Build history of the part. All positions in model axes, mm. A direction names the side the tool comes from. Round coordinates to 2 decimals unless told otherwise and drop trailing zeros. Write each loop counter-clockwise with the first axis right and the second up, starting at its lowest first coordinate (ties: lowest second). Pieces come first, ordered by that corner, then holes. Notation, with made-up numbers: (28.5, 10.25) - (60.5, 10.25) arc R14 cw to (60.5, 14.25) - close; hole circle Ø8 at (81, 77). An arc over 180 degrees is marked (long way). Answer as a JSON object with one key per item and string values. Group by question number.
Item 1: Probe line 1 (Z direction, x = 22.5, y = 9.1); line 2 (Y direction, x = 26.25, z = -27) (3 decimals); line 3 (Z direction, x = 23.5, y = 8.5). List the from-to ranges inside material, lowest first. Write a range as from..to.
Item 2: Two-plate mould, pull along Y, no slides. Class faces 4 (the flat face through (23.946, 16.896, -28.319)), 5 (the cylindrical face through (23.95, 10.18, -28.18)), 6 (the flat face through (24, 9, -35)): +Y half, -Y half, draft (parallel to the pull), parting line (faces both ways), or undercut.
Item 3: Flat gauge pin, fed straight in: pin 1 (0.7 mm diameter, centred on x = 22.5, z = -35, fed in from +Y). Where does the tip first touch, or does it go through?
Item 4: Slice it at A-A, the plane z = -27. List the corners of the cut face in (x, y) (3 decimals), then the cut area to 3 significant figures.
Item 5: Which spindle directions (+Z, -Z, +X, -X, +Y, -Y) get a long thin tool onto all of the face, cutting with end or side? Do faces 1 (the flat face through (23.946, 16.896, -18.894)), 2 (the flat face through (24.1, 15, -34.6)), 3 (the cylindrical face through (23.95, 10.18, -8.18)). Say none if no direction does.
Item 6: Slice it at C-C, the plane y = 16.5. Give the number of separate pieces and of enclosed holes in the cut face, then the cut area to 3 significant figures.
Item 7: Slice it at B-B, the plane y = 9.1. List the corners of the cut face in (x, z) (3 decimals), then the cut area to 3 significant figures.
from build123d import *

# Parameters (mm, degrees)
ESQUISSE1_W                 = 24
ESQUISSE1_H                 = 30
MAIN_EXTRUSION_DEPTH        = 30
MAIN_RIDING_HOLE_DEPTH      = 31
ESQUISSE4_R                 = 2.25
TRACTORHOLE_DEPTH           = 8
IMPACTPIECE_DEPTH           = 4.5
CONG_1_R                    = 3
TEETH_DEPTH                 = 4.5
CONG_3_R                    = 0.57
TEETHREPETITION_COUNT       = 8
TEETHREPETITION_PITCH       = 4.71238898
CONG_3_OF_TEETHREPETITION_R = 0.57
ESQUISSE9_W                 = 55
ESQUISSE9_H                 = 15.375
BRACKET_DEPTH               = 0.675
BRACKETHOLE_START           = -8.5
ESQUISSE10_R                = 1.6
BRACKETHOLE_DEPTH           = 26
BRACKETHOLEREPETITION_COUNT = 5
BRACKETHOLEREPETITION_PITCH = 10
ESQUISSE11_W                = 7.5
ESQUISSE11_H                = 5.5
ESQUISSE11_H_2              = 7.6
RAILHOLE_DEPTH              = 20
TOPIMPACTCUT_DEPTH          = 17.5
ESQUISSE13_W                = 24
ESQUISSE13_H                = 50
MAKERBEAMMAINHOLE_DEPTH     = 81
SKETCH1_W                   = 24
SKETCH1_H                   = 45
KEEPONLYTRACTOR1_DEPTH      = 51


with BuildPart() as part:
    # Esquisse1 → Main Extrusion (new body)
    with BuildSketch(Plane.XY):
        Rectangle(ESQUISSE1_W, ESQUISSE1_H)
    extrude(amount=MAIN_EXTRUSION_DEPTH)

    # Esquisse3 → Main Riding Hole (cut, through all)
    with BuildSketch(Plane(origin=(0, 0, 0), x_dir=(-1, 0, 0), z_dir=(0, 0, -1))):
        Polygon((-5.2, -1.6), (-5.2, -5.4), (-4.2, -5.4), (-4.2, -8.2), (-5.2, -8.2), (-5.2, -12), (-1.4, -12), (-1.4, -11), (1.4, -11), (1.4, -12), (5.2, -12), (5.2, -8.2), (4.2, -8.2), (4.2, -5.4), (5.2, -5.4), (5.2, -1.6), (1.4, -1.6), (1.4, -2.6), (-1.4, -2.6), (-1.4, -1.6), align=None)
    extrude(amount=-MAIN_RIDING_HOLE_DEPTH, mode=Mode.SUBTRACT)

    # Esquisse4 → TractorHole (cut)
    with BuildSketch(Plane.ZY.offset(12)):
        with Locations((5, -6.8)):
            Circle(ESQUISSE4_R)
    tractorhole = extrude(amount=-TRACTORHOLE_DEPTH, mode=Mode.SUBTRACT)

    # TractorHoleSymetry: TractorHole across plane
    add(tractorhole.mirror(Plane(origin=(0, 0, 0), x_dir=(0, 0, 1), z_dir=(1, 0, 0))), mode=Mode.SUBTRACT)

    # Esquisse5 → ImpactPiece (add, symmetric)
    with BuildSketch(Plane(origin=(0, 0, 0), x_dir=(0, 0, -1), z_dir=(1, 0, 0))):
        Polygon((-45, 5), (-45, 35), (-25, 35), (-21.473460386, 15), (35, 15), (35, 3), (0, 3), (0, 5), align=None)
    extrude(amount=IMPACTPIECE_DEPTH, both=True)

    # Congé1
    cong_1_edges = [part.edges().sort_by_distance(p)[0] for p in [
        (4.5, 15, 25.736730193),
        (-4.5, 15, 25.736730193),
    ]]
    fillet(cong_1_edges, radius=CONG_1_R)

    # Esquisse8 → Teeth (add, symmetric)
    with BuildSketch(Plane(origin=(0, 0, 0), x_dir=(0, 0, -1), z_dir=(1, 0, 0))):
        Polygon((30, 15), (31.228399541, 18.375), (32.492683328, 18.375), (33.721082869, 15), align=None)
    teeth = extrude(amount=TEETH_DEPTH, both=True)

    # Congé3
    cong_3_edges = [part.edges().sort_by_distance(p)[0] for p in [
        (0, 15, -30),
        (0, 15, -33.721082869),
    ]]
    fillet(cong_3_edges, radius=CONG_3_R)

    # TeethRepetition: Teeth ×8
    with Locations(*[(0, 0, i * TEETHREPETITION_PITCH) for i in range(1, TEETHREPETITION_COUNT)]):
        add(teeth)

    # Congé3 of TeethRepetition
    cong_3_of_teethrepetition_edges = [part.edges().sort_by_distance(p)[0] for p in [
        (0, 15, -25.28761102),
        (0, 15, -29.008693889),
        (0, 15, -20.57522204),
        (0, 15, -24.296304909),
        (0, 15, -15.86283306),
        (0, 15, -19.583915929),
        (0, 15, -11.15044408),
        (0, 15, -14.871526949),
        (0, 15, -6.4380551),
        (0, 15, -10.159137969),
        (0, 15, -1.72566612),
        (0, 15, -5.446748989),
        (0, 15, 2.98672286),
        (0, 15, -0.734360009),
    ]]
    fillet(cong_3_of_teethrepetition_edges, radius=CONG_3_OF_TEETHREPETITION_R)

    # Esquisse9 → Bracket (cut, symmetric)
    with BuildSketch(Plane(origin=(4.5, 0, 0), x_dir=(0, 0, -1), z_dir=(1, 0, 0))):
        with Locations((7.5, 10.6875)):
            Rectangle(ESQUISSE9_W, ESQUISSE9_H)
    bracket = extrude(amount=BRACKET_DEPTH, both=True, mode=Mode.SUBTRACT)

    # Esquisse10 → BracketHole (cut)
    with BuildSketch(Plane.ZY.offset(-4.5).offset(BRACKETHOLE_START)):
        with Locations((-27, 9.1)):
            Circle(ESQUISSE10_R)
    brackethole = extrude(amount=BRACKETHOLE_DEPTH, mode=Mode.SUBTRACT)

    # BracketHoleRepetition: BracketHole ×5
    with Locations(*[(0, 0, i * BRACKETHOLEREPETITION_PITCH) for i in range(1, BRACKETHOLEREPETITION_COUNT)]):
        add(brackethole, mode=Mode.SUBTRACT)

    # Symétrie1: Bracket across plane
    add(bracket.mirror(Plane(origin=(0, 0, 0), x_dir=(0, 0, 1), z_dir=(1, 0, 0))), mode=Mode.SUBTRACT)

    # Esquisse11 → RailHole (cut)
    with BuildSketch(Plane(origin=(0, 0, 0), x_dir=(-1, 0, 0), z_dir=(0, 0, -1))):
        with Locations((8.25, 3.15)):
            Rectangle(ESQUISSE11_W, ESQUISSE11_H)
        with Locations((8.25, 16.2)):
            Rectangle(ESQUISSE11_W, ESQUISSE11_H_2)
    extrude(amount=-RAILHOLE_DEPTH, mode=Mode.SUBTRACT)

    # Esquisse12 → TopImpactCut (cut, through all)
    with BuildSketch(Plane(origin=(4.5, 0, 0), x_dir=(0, 0, -1), z_dir=(1, 0, 0))):
        Polygon((-45, 30), (-40, 35), (-45, 35), align=None)
    extrude(amount=-TOPIMPACTCUT_DEPTH, mode=Mode.SUBTRACT)


with BuildPart() as body_2:
    # Symétrie2: mirrored copy
    add(part.part.mirror(Plane(origin=(12, 15, 30), x_dir=(0, 0, 1), z_dir=(-1, 0, 0))))

    # Sketch1 → KeepOnlyTractor1 (cut, through all)
    with BuildSketch(Plane(origin=(0, 35, 0), x_dir=(1, 0, 0), z_dir=(0, 1, 0))):
        with Locations((24, -22.5)):
            Rectangle(SKETCH1_W, SKETCH1_H)
    extrude(amount=-KEEPONLYTRACTOR1_DEPTH, mode=Mode.SUBTRACT)


with BuildPart() as part_1:
    add(part.part)

    # Esquisse13 → MakerBeamMainHole (cut, through all)
    with BuildSketch(Plane(origin=(0, 0, -35), x_dir=(-1, 0, 0), z_dir=(0, 0, -1))):
        with Locations((0, 10)):
            Rectangle(ESQUISSE13_W, ESQUISSE13_H)
    extrude(amount=-MAKERBEAMMAINHOLE_DEPTH, mode=Mode.SUBTRACT)


solid = body_2.part
Geometry says:
{
 "1": {"line 1": "z = -35..-28.6, -25.4..-18.6, -15.4..-8.6, -5.4..0", "line 2": "y = 3..7.5, 10.7..18.375", "line 3": "z = -35..-28.48, -25.52..-18.48, -15.52..-8.48, -5.52..0"},
 "2": {"face 4": "+Y half", "face 5": "undercut", "face 6": "draft"},
 "3": {"pin 1": "stops at y = 15"},
 "4": {"outline": "(20.175, 3) - (27.825, 3) - (27.825, 7.5) - (20.175, 7.5) - close; (20.175, 10.7) - (27.825, 10.7) - (27.825, 18.375) - (20.175, 18.375) - close", "area": "93.1 mm^2"},
 "5": {"face 1": "+X, -X, +Y", "face 2": "-Z, +X, -X, +Y", "face 3": "+X, -X"},
 "6": {"separate pieces": "8", "enclosed holes": "0", "area": "142 mm^2"},
 "7": {"outline": "(20.175, -35) - (27.825, -35) - (27.825, -28.6) - (20.175, -28.6) - close; (20.175, -25.4) - (27.825, -25.4) - (27.825, -18.6) - (20.175, -18.6) - close; (20.175, -15.4) - (27.825, -15.4) - (27.825, -8.6) - (20.175, -8.6) - close; (20.175, -5.4) - (27.825, -5.4) - (27.825, 0) - (20.175, 0) - close", "area": "194 mm^2"}
}
